The model under review builds one solid part; all positions refer to its coordinate system, in mm. A direction names the side the tool comes from. Coordinates: 2 decimals unless noted, no trailing zeros. Write each loop counter-clockwise with the first axis right and the second up, starting at its lowest first coordinate (ties: lowest second). Pieces come first, ordered by that corner, then holes. Notation, with made-up numbers: (-18.75, -28.75) - (3.25, -28.75) arc R31 cw to (3.25, -2.75) - close; hole circle Ø3 at (24, 24.25). An arc over 180 degrees is marked (long way). Put each result on its own line as item: value.
from build123d import *

# Parameters (mm, degrees)
F0_W     = 200
F0_H     = 49.526437
F1_DEPTH = 10
F2_R     = 5
F3_R     = 5
F3_R_2   = 10
F4_DEPTH = 10.001
F5_W     = 50
F5_H     = 20
F6_DEPTH = 25


with BuildPart() as f1:
    # F0 (on Top) → F1 (new body)
    with BuildSketch(Plane.XY):
        with Locations((-52.009064, -0.236782)):
            Rectangle(F0_W, F0_H)
    extrude(amount=F1_DEPTH)

    # F2
    f2_edges = [f1.edges().sort_by_distance(p)[0] for p in [
        (47.990936, -25, 5),
        (47.990936, 24.526437, 5),
        (-152.009064, -25, 5),
        (-152.009064, 24.526437, 5),
    ]]
    fillet(f2_edges, radius=F2_R)

    # F3 (on face) → F4 (cut, through all)
    with BuildSketch(Plane.XY.offset(10)):
        with Locations((-52.009064, 0)):
            Circle(F3_R)
        with Locations((-102.009064, 0)):
            Circle(F3_R_2)
    extrude(amount=-F4_DEPTH, mode=Mode.SUBTRACT)

    # F5 (on face) → F6 (cut)
    with BuildSketch(Plane.XY.offset(10)):
        with Locations((22.990936, 0)):
            Rectangle(F5_W, F5_H)
    extrude(amount=-F6_DEPTH, mode=Mode.SUBTRACT)


solid = f1.part
1. To check wall thickness, follow probe 1 along X at (y, z) = (-1, 4.25); probe 2 along Y at (x, z) = (21.5, 2.75); probe 3 along X at (y, z) = (-6.5, 4). State the ranges of each line that lie inside material, in increasing order.
Determined:
probe 1: x = -152.01 to -111.96, -92.06 to -56.91, -47.11 to -2.01
probe 2: y = -25 to -10, 10 to 24.53
probe 3: x = -152.01 to -109.61, -94.41 to -2.01
2. The part is to be moulded in two halves that separate along X. For faces 3 (the cylindrical face through (-150.58, -23.5, 5.07)), 4 (the cylindrical face through (-92.77, -3.83, 5.07)), 5 (the flat face through (23, -10, 5)), say which applies: +X half, -X half, draft (parallel to the pull), parting line (faces both ways), or undercut.
Determined:
face 3: -X half
face 4: undercut
face 5: draft
3. Consider section C-C on z = 8. State the section outline as (x, y) points, plus the area to 3 significant figures.
Determined:
outline: (-152.01, -20) arc R5 ccw to (-147.01, -25) - (42.99, -25) arc R5 ccw to (47.99, -20) - (47.99, -10) - (-2.01, -10) - (-2.01, 10) - (47.99, 10) - (47.99, 19.53) arc R5 ccw to (42.99, 24.53) - (-147.01, 24.53) arc R5 ccw to (-152.01, 19.53) - close; hole circle Ø20 at (-102.01, 0); hole circle Ø10 at (-52.01, 0)
area: 8,490 mm^2
4. Consider section A-A on x = 9. State the section outline as (y, z) points, plus the area to 3 significant figures.
Determined:
outline: (-25, 0) - (-10, 0) - (-10, 10) - (-25, 10) - close; (10, 0) - (24.53, 0) - (24.53, 10) - (10, 10) - close
area: 295 mm^2
5. Machinability: for faces 1 (the flat face through (47.991, 15, 5)), 2 (the flat face through (-2.009, 0, 5)), which of the approach directions +Z, -Z, +X, -X, +Y, -Y give a long, thin tool a straight path to every point of the face, cutting with its end or side? Answer none if there is none.
Determined:
face 1: +Z, -Z, +X, +Y, -Y
face 2: +Z, -Z, +X
6. Consider section B-B on y = 0. State the section outline as (x, z) points.
Determined:
outline: (-152.01, 0) - (-112.01, 0) - (-112.01, 10) - (-152.01, 10) - close; (-92.01, 0) - (-57.01, 0) - (-57.01, 10) - (-92.01, 10) - close; (-47.01, 0) - (-2.01, 0) - (-2.01, 10) - (-47.01, 10) - close
7. Consider section D-D on x = -109. State the section outline as (y, z) points, plus the area to 3 significant figures.
Determined:
outline: (-25, 0) - (-7.15, 0) - (-7.15, 10) - (-25, 10) - close; (7.15, 0) - (24.53, 0) - (24.53, 10) - (7.15, 10) - close
area: 352 mm^2
